from build123d import *

# Parameters (mm, degrees)
PAD_DEPTH       = 20
SKETCH006_R     = 10
POCKET_DEPTH    = 20.001
SKETCH005_R     = 11.05
POCKET001_DEPTH = 7
SKETCH002_R     = 2.25
POCKET002_DEPTH = 65.001
SKETCH003_R     = 5
POCKET003_DEPTH = 5
SKETCH007_R     = 2.25
POCKET004_DEPTH = 70.001
SKETCH008_R     = 5
POCKET005_DEPTH = 5
SKETCH009_R     = 11.05
POCKET006_DEPTH = 7
SKETCH010_R     = 6.05
POCKET007_DEPTH = 20.001
SKETCH011_W     = 1
SKETCH011_H     = 25
POCKET008_DEPTH = 20.001
SKETCH012_R     = 1.25
POCKET009_DEPTH = 20.001


with BuildPart() as part:
    # Sketch → Pad (new body)
    with BuildSketch(Plane.XY):
        with BuildLine():
            Line((-35, 22), (35, 22))
            Line((35, -43), (35, 22))
            Line((6, -43), (35, -43))
            Line((6, -43), (6, -19.078784))
            ThreePointArc((-20, 0), (-11.83216, -16.124515), (6, -19.078784))
            Line((-20, 0), (-20, 7))
            Line((-20, 7), (-35, 7))
            Line((-35, 7), (-35, 22))
        make_face()
    extrude(amount=PAD_DEPTH)

    # Sketch006 → Pocket (cut, through all)
    with BuildSketch(Plane(origin=(0, 0, 0), x_dir=(1, 0, 0), z_dir=(0, 0, -1))):
        Circle(SKETCH006_R)
    extrude(amount=-POCKET_DEPTH, mode=Mode.SUBTRACT)

    # Sketch005 → Pocket001 (cut)
    with BuildSketch(Plane.XY.offset(20)):
        Circle(SKETCH005_R)
    extrude(amount=-POCKET001_DEPTH, mode=Mode.SUBTRACT)

    # Sketch002 → Pocket002 (cut, through all)
    with BuildSketch(Plane(origin=(0, 22, 0), x_dir=(-1, 0, 0), z_dir=(0, 1, 0))):
        with Locations((27.5, 10)):
            Circle(SKETCH002_R)
    extrude(amount=-POCKET002_DEPTH, mode=Mode.SUBTRACT)

    # Sketch003 → Pocket003 (cut)
    with BuildSketch(Plane.XZ.offset(-7)):
        with Locations((-27.5, 10)):
            Circle(SKETCH003_R)
    extrude(amount=-POCKET003_DEPTH, mode=Mode.SUBTRACT)

    # Sketch007 → Pocket004 (cut, through all)
    with BuildSketch(Plane.YZ.offset(35)):
        with Locations((-32, 10)):
            Circle(SKETCH007_R)
    extrude(amount=-POCKET004_DEPTH, mode=Mode.SUBTRACT)

    # Sketch008 → Pocket005 (cut)
    with BuildSketch(Plane(origin=(6, 0, 0), x_dir=(0, -1, 0), z_dir=(-1, 0, 0))):
        with Locations((32, 10)):
            Circle(SKETCH008_R)
    extrude(amount=-POCKET005_DEPTH, mode=Mode.SUBTRACT)

    # Sketch009 → Pocket006 (cut)
    with BuildSketch(Plane(origin=(0, 0, 0), x_dir=(1, 0, 0), z_dir=(0, 0, -1))):
        Circle(SKETCH009_R)
    extrude(amount=-POCKET006_DEPTH, mode=Mode.SUBTRACT)

    # Sketch010 → Pocket007 (cut, through all)
    with BuildSketch(Plane.XY.offset(20)):
        with Locations((20, -23)):
            Circle(SKETCH010_R)
    extrude(amount=-POCKET007_DEPTH, mode=Mode.SUBTRACT)

    # Sketch011 → Pocket008 (cut, through all)
    with BuildSketch(Plane.XY.offset(20)):
        with Locations((20, -32.5)):
            Rectangle(SKETCH011_W, SKETCH011_H)
    extrude(amount=-POCKET008_DEPTH, mode=Mode.SUBTRACT)

    # Sketch012 → Pocket009 (cut, through all)
    with BuildSketch(Plane.XY.offset(20)):
        with Locations((9.545942, 9.545942)):
            Circle(SKETCH012_R)
        with Locations((-13.039999, 3.494057)):
            Circle(SKETCH012_R)
        with Locations((3.494057, -13.039999)):
            Circle(SKETCH012_R)
    extrude(amount=-POCKET009_DEPTH, mode=Mode.SUBTRACT)


solid = part.part
For this review, take the finished solid that the model builds, in its own axes (mm). A direction names the side the tool comes from. Round coordinates to 2 decimals unless told otherwise and drop trailing zeros. Order: outer loops, then holes, each group sorted by start corner. A loop starts at its lowest first (then second) coordinate and runs counter-clockwise, first axis right, second up. Notation, with made-up numbers: (55.25, 36) -> (79.25, 36) arc R17 ccw to (79.25, 41) -> close; hole circle Ø3 at (-37.5, -26.5). An arc over 180 degrees is marked (long way). Put each result on its own line as item: value.
Q1. Insertion check: pin 1 Ø7.5 at (x, z) = (-25.5, 9) entering from -Y; pin 2 Ø2 at (x, y) = (-6.5, 10) entering from -Z; pin 3 Ø3.5 at (y, z) = (5, 8.5) entering from -X; pin 4 Ø5 at (x, z) = (-28.5, 9) entering from -Y. Each pin has a flat end and moves straight along its axis. Give the tip position at first contact, or say it passes through.
Check result:
pin 1: y = 7
pin 2: z = 0
pin 3: x = -20
pin 4: y = 12
Q2. Add section D-D on x = -27.5. Write out the cut boundary in (y, z).
Check result:
outline: (7, 0) -> (22, 0) -> (22, 7.75) -> (12, 7.75) -> (12, 5) -> (7, 5) -> close; (7, 15) -> (12, 15) -> (12, 12.25) -> (22, 12.25) -> (22, 20) -> (7, 20) -> close
Q3. For probe 1 along X at (y, z) = (9.5, 3.25); probe 2 along Y at (x, z) = (22.5, 10.75); probe 3 along Y at (x, z) = (0, 2), list the stretches that pass through material, from the lowest coordinate up. Write a range as [from, to].
Check result:
probe 1: [-35, -5.64], [5.64, 8.3], [10.8, 35]
probe 2: [-43, -34.12], [-29.88, -28.51], [-17.49, 22]
probe 3: [-20, -11.05], [11.05, 22]
Q4. Add section A-A on x = 0. Write out the cut boundary in (y, z), plus the area to 3 significant figures.
Check result:
outline: (-20, 0) -> (-11.05, 0) -> (-11.05, 7) -> (-10, 7) -> (-10, 13) -> (-11.05, 13) -> (-11.05, 20) -> (-20, 20) -> close; (10, 7) -> (11.05, 7) -> (11.05, 0) -> (22, 0) -> (22, 20) -> (11.05, 20) -> (11.05, 13) -> (10, 13) -> close
area: 411 mm2
Q5. Mouldability with a two-part tool opening along Y and no side actions: class faces 1 (the flat face through (-22, 7, 10)), 2 (the flat face through (8, -10, 20)), 3 (the cylindrical face through (-2.17, 9.76, 9.96)), 4 (the cylindrical face through (4.07, -14.15, 10.14)) as pulls with the +Y half, pulls with the -Y half, needs draft (parallel to the pull), parting line crosses it, or undercut.
Check result:
face 1: pulls with the -Y half
face 2: needs draft
face 3: undercut
face 4: undercut
Q6. Machinability: for faces 5 (the flat face through (-26, 12, 8)), 6 (the flat face through (19.5, -36, 10)), 7 (the flat face through (11, -33, 7.8)), which of the approach directions +Z, -Z, +X, -X, +Y, -Y give a long, thin tool a straight path to every point of the face, cutting with its end or side? Answer none if there is none.
Check result:
face 5: -Y
face 6: +Z, -Z, -Y
face 7: -X
Q7. Add section B-B on y = -32. Write out the cut boundary in (x, z).
Check result:
outline: (6, 0) -> (19.5, 0) -> (19.5, 7.75) -> (11, 7.75) -> (11, 5) -> (6, 5) -> close; (6, 15) -> (11, 15) -> (11, 12.25) -> (19.5, 12.25) -> (19.5, 20) -> (6, 20) -> close; (20.5, 0) -> (35, 0) -> (35, 7.75) -> (20.5, 7.75) -> close; (20.5, 12.25) -> (35, 12.25) -> (35, 20) -> (20.5, 20) -> close
Q8. Add section C-C on z = 10. State how many separate pieces and enclosed holes the cut face has, plus the area to 3 significant figures.
Check result:
separate pieces: 4
enclosed holes: 4
area: 2,410 mm2
